Drawing for the job (mm, zero at the part's lowest x, y, z). Coordinates: 2 decimals unless noted, no trailing zeros. Order: outer loops, then holes, each group sorted by start corner. A loop starts at its lowest first (then second) coordinate and runs counter-clockwise, first axis right, second up.
1) Cut at A-A (z = 16.75). List the corners of the cut face in (x, y) (1 decimal).
2) Wall check: L1, parallel to Z at x = 17.5, y = 2; L2, parallel to X at y = 11, z = 10 (1 decimal); L3, parallel to X at y = 18, z = 11.75. Give the ranges that are in metal, low to high.
3) Mould opens along X. For the marked faces 1, 2 and 3 say: +X half, -X half, draft (parallel to the pull), parting line (faces both ways), or undercut.
4) Pin check, flat tips, straight feed: pin 1 Ø1 at (x, z) = (12.5, 18) entering from -Y (1 decimal); pin 2 Ø12 at (x, z) = (28, 4) entering from +Y (1 decimal); pin 3 Ø1.5 at (y, z) = (26, 21.5) entering from +X. Stop position of each tip, or through.
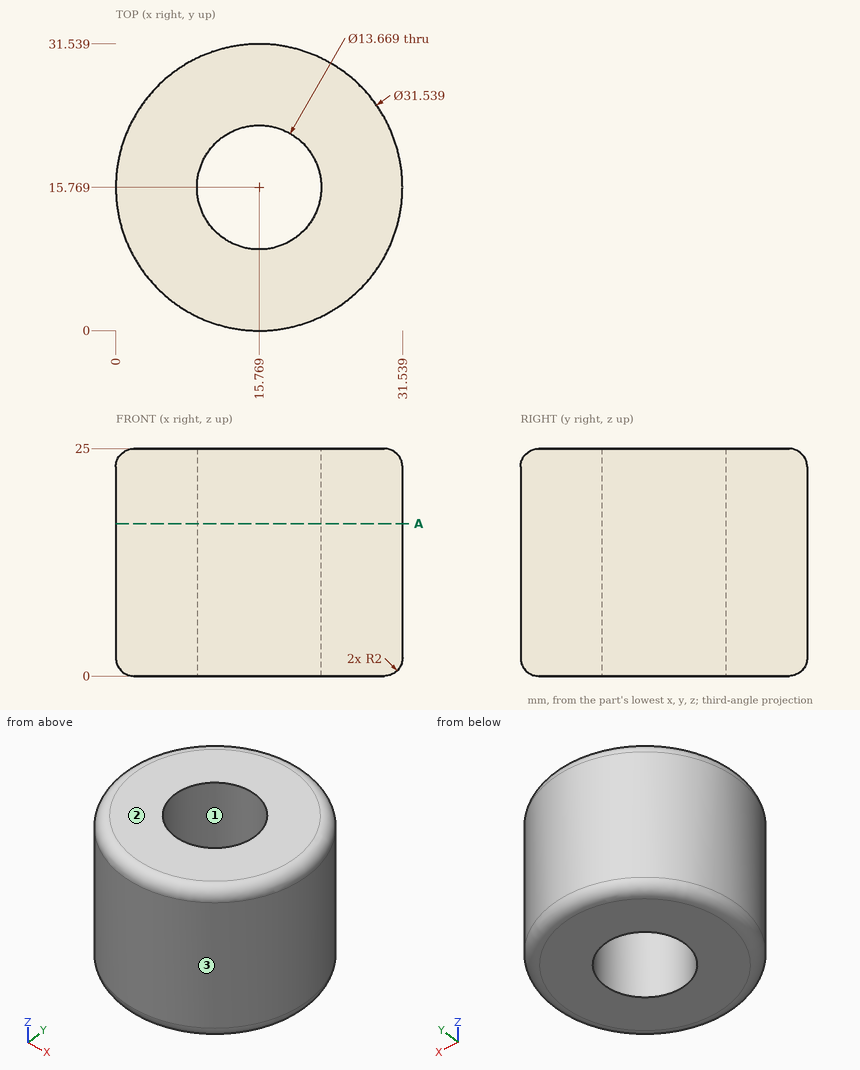
Geometry check:
1. outline: circle Ø31.5 at (15.8, 15.8); hole circle Ø13.7 at (15.8, 15.8)
2. L1: z = 0 to 25
2. L2: x = 0.7 to 10.9, 20.7 to 30.8
2. L3: x = 0.16 to 9.31, 22.23 to 31.38
3. face 1: undercut
3. face 2: draft
3. face 3: parting line
4. pin 1: stops at y = 0.2
4. pin 2: stops at y = 30.3
4. pin 3: stops at x = 28.37
